Geometry: see drawing. Coordinates: mm, zero at the bounding-box minimum. Give positions to 0.01 mm unless a question says otherwise; leave off trailing zeros. Loops run counter-clockwise (first coordinate to the right, second up) from the corner with the lowest first, then second, coordinate; pieces in that order, holes last. Notation, with made-up numbers: (35.25, -32) -> (39.25, -32) arc R11 ccw to (39.25, -26) -> close; hole circle Ø10 at (-20.5, 45.25). An arc over 180 degrees is marked (long way). Return JSON: item names as keys, results as strings. Group by question number.
(1) Cut plane D-D on x = 6.25. Return loops of the section in (y, z).
(2) Cut plane B-B on z = 4.35. Return loops of the section in (x, y), then the cut area to 3 significant figures.
(3) Cut plane A-A on z = 1.25. Return loops of the section in (x, y), then the cut area to 3 significant figures.
(4) Ray query, line 1 (X direction, y = 0.05, z = 1.65); line 2 (X direction, y = 0.05, z = 2.25); line 3 (Z direction, x = 4.5, y = 0.05). Return the intervals inside material, ascending. Write a range as from..to.
(5) Cut plane C-C on y = 0.05. Return loops of the section in (x, z).
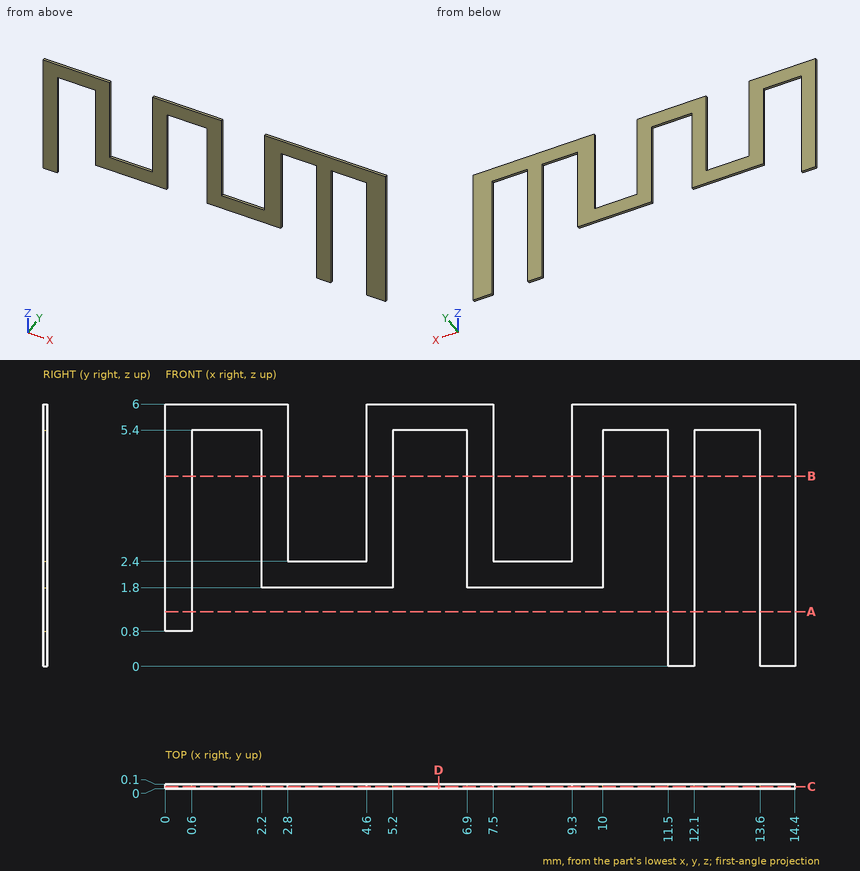
Answers:
{
 "1": {"outline": "(0, 5.4) -> (0.1, 5.4) -> (0.1, 6) -> (0, 6) -> close"},
 "2": {"outline": "(0, 0) -> (0.6, 0) -> (0.6, 0.1) -> (0, 0.1) -> close; (2.2, 0) -> (2.8, 0) -> (2.8, 0.1) -> (2.2, 0.1) -> close; (4.6, 0) -> (5.2, 0) -> (5.2, 0.1) -> (4.6, 0.1) -> close; (6.9, 0) -> (7.5, 0) -> (7.5, 0.1) -> (6.9, 0.1) -> close; (9.3, 0) -> (10, 0) -> (10, 0.1) -> (9.3, 0.1) -> close; (11.5, 0) -> (12.1, 0) -> (12.1, 0.1) -> (11.5, 0.1) -> close; (13.6, 0) -> (14.4, 0) -> (14.4, 0.1) -> (13.6, 0.1) -> close", "area": "0.450 mm²"},
 "3": {"outline": "(0, 0) -> (0.6, 0) -> (0.6, 0.1) -> (0, 0.1) -> close; (11.5, 0) -> (12.1, 0) -> (12.1, 0.1) -> (11.5, 0.1) -> close; (13.6, 0) -> (14.4, 0) -> (14.4, 0.1) -> (13.6, 0.1) -> close", "area": "0.200 mm²"},
 "4": {"line 1": "0..0.6, 11.5..12.1, 13.6..14.4", "line 2": "0..0.6, 2.2..5.2, 6.9..10, 11.5..12.1, 13.6..14.4", "line 3": "1.8..2.4"},
 "5": {"outline": "(0, 0.8) -> (0.6, 0.8) -> (0.6, 5.4) -> (2.2, 5.4) -> (2.2, 1.8) -> (5.2, 1.8) -> (5.2, 5.4) -> (6.9, 5.4) -> (6.9, 1.8) -> (10, 1.8) -> (10, 5.4) -> (11.5, 5.4) -> (11.5, 0) -> (12.1, 0) -> (12.1, 5.4) -> (13.6, 5.4) -> (13.6, 0) -> (14.4, 0) -> (14.4, 6) -> (9.3, 6) -> (9.3, 2.4) -> (7.5, 2.4) -> (7.5, 6) -> (4.6, 6) -> (4.6, 2.4) -> (2.8, 2.4) -> (2.8, 6) -> (0, 6) -> close"}
}
